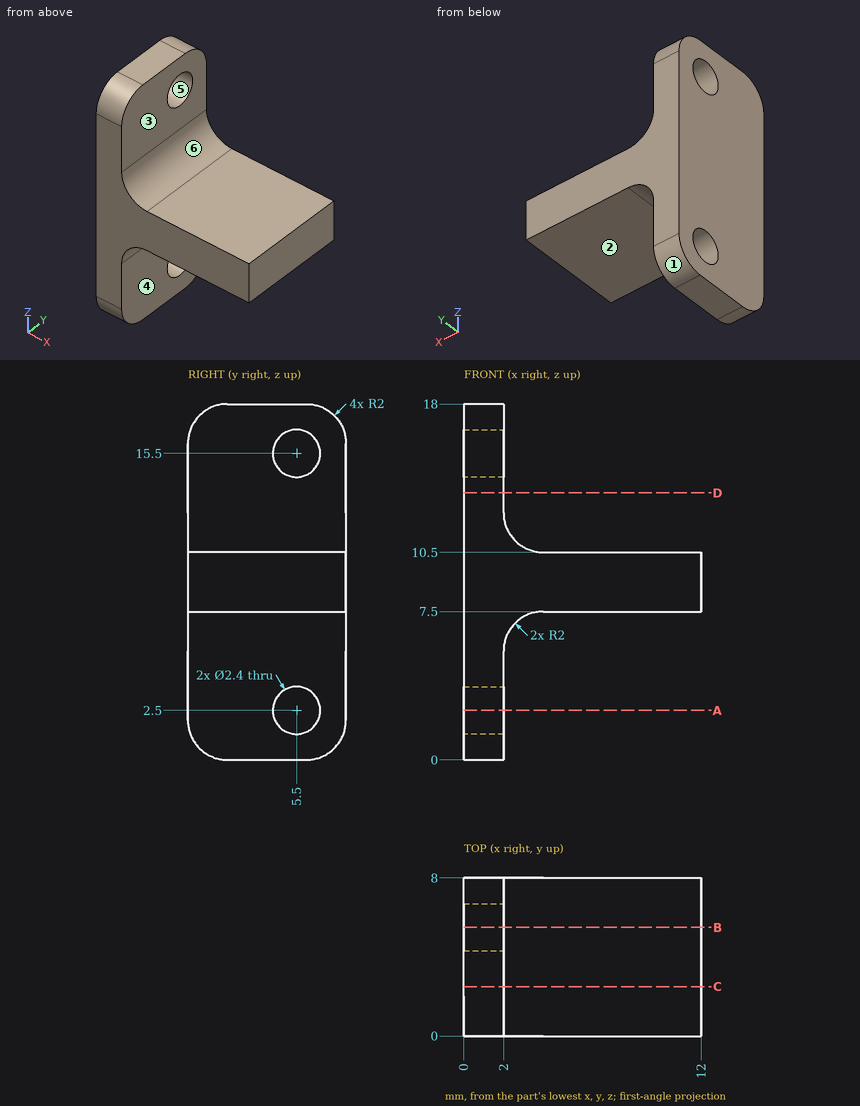
Source: three-view drawing plus pictorial views. Frame: mm from the lowest corner of the part. A direction names the side the tool comes from. Round coordinates to 2 decimals unless told otherwise and drop trailing zeros. Loops run counter-clockwise (first coordinate to the right, second up) from the corner with the lowest first, then second, coordinate; pieces in that order, holes last. Notation, with made-up numbers: (28.25, 10.25) - (52.25, 10.25) arc R14 cw to (52.25, 19.25) - close; hole circle Ø10 at (-19, 40.25). An arc over 180 degrees is marked (long way). Write item = value, one per line. Start each with the question number.
Item 1: Section query B-B on y = 5.5. Output: boundary loops of the cut face in (x, z), plus the area to 3 significant figures.
Item 2: Reachability of the marked faces 1, 2 and 3 from +Z, -Z, +X, -X, +Y, -Y: full face, straight path, thin tool, end or side. Return the list, or none.
Item 3: Section query C-C on y = 2.5. Output: boundary loops of the cut face in (x, z), plus the area to 3 significant figures.
Item 4: Material intervals for line 1 (Y direction, x = 0.85, z = 2.5); line 2 (X direction, y = 6, z = 4); line 3 (Z direction, x = 6, y = 5.75), sorted ascending.
Item 5: Section query D-D on z = 13.5. Output: boundary loops of the cut face in (x, y), plus the area to 3 significant figures.
Item 6: First-contact query: pin 1 Ø4.5 at (y, z) = (4.5, 3.5) entering from +X; pin 2 Ø2 at (x, y) = (8, 6.5) entering from +Z. Flat tips, straight axial feed; report the tip coordinate or a pass-through.
Item 7: Mould query, pull axis Z, two halves, no side actions, for the marked faces 4, 5 and 6. Classes: released by +Z, released by -Z, zero draft, split by the parting line, or undercut.
Item 8: Section query A-A on z = 2.5. Output: boundary loops of the cut face in (x, y).
Results list:
q1.outline = (0, 0) - (2, 0) - (2, 1.3) - (0, 1.3) - close; (0, 3.7) - (2, 3.7) - (2, 5.5) arc R2 cw to (4, 7.5) - (12, 7.5) - (12, 10.5) - (4, 10.5) arc R2 cw to (2, 12.5) - (2, 14.3) - (0, 14.3) - close; (0, 16.7) - (2, 16.7) - (2, 18) - (0, 18) - close
q1.area = 58.1 mm²
q2.face_1 = -Z, +X, -X, +Y
q2.face_2 = -Z, +X, +Y, -Y
q2.face_3 = +Z, +X, +Y, -Y
q3.outline = (0, 0) - (2, 0) - (2, 5.5) arc R2 cw to (4, 7.5) - (12, 7.5) - (12, 10.5) - (4, 10.5) arc R2 cw to (2, 12.5) - (2, 18) - (0, 18) - close
q3.area = 67.7 mm²
q4.line_1 = 0 to 4.3, 6.7 to 8
q4.line_2 = 0 to 2
q4.line_3 = 7.5 to 10.5
q5.outline = (0, 0) - (2, 0) - (2, 8) - (0, 8) - close
q5.area = 16.0 mm²
q6.pin_1 = 2.02
q6.pin_2 = 10.5
q7.face_4 = zero draft
q7.face_5 = undercut
q7.face_6 = released by +Z
q8.outline = (0, 0) - (2, 0) - (2, 4.3) - (0, 4.3) - close; (0, 6.7) - (2, 6.7) - (2, 8) - (0, 8) - close
